Design review of the part built by this model. Coordinates are the model's own, in mm. Coordinates: 2 decimals unless noted, no trailing zeros. Loops run counter-clockwise (first coordinate to the right, second up) from the corner with the lowest first, then second, coordinate; pieces in that order, holes last. Notation, with made-up numbers: M -18.5,-37.5 L 6.5,-37.5 A12 ccw 6.5,-27.5 Z; hole C -33,-35.75 d8. An arc over 180 degrees is marked long. One line per item, written item: value.
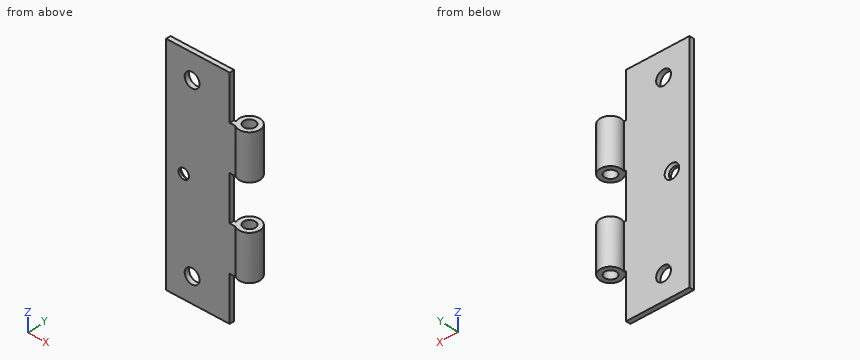
```python
from build123d import *

# Parameters (mm, degrees)
BOSS_EXTRUDE1_DEPTH                            = 15.24
SKETCH2_W                                      = 15.24
SKETCH2_H                                      = 1.5748
BOSS_EXTRUDE2_DEPTH                            = 0.254646985
SKETCH3_W                                      = 30.48
SKETCH3_H                                      = 1.5748
BOSS_EXTRUDE3_DEPTH                            = 21.866377542
SKETCH4_W                                      = 15.24
SKETCH4_H                                      = 1.5748
CUT_EXTRUDE1_DEPTH                             = 0.403377542
BOSS_EXTRUDE4_DEPTH                            = 15.24
SKETCH6_W                                      = 21.463
SKETCH6_H                                      = 1.5748
BOSS_EXTRUDE5_DEPTH                            = 15.24
SKETCH7_W                                      = 21.463
SKETCH7_H                                      = 1.5748
BOSS_EXTRUDE6_DEPTH                            = 15.24
SKETCH8_W                                      = 1.984375
SKETCH8_H                                      = 30.480025
M3_5_CLEARANCE_HOLE2_D                         = 3.96875
M3_5_CLEARANCE_HOLE2_DEPTH                     = 60.960025
CSK_FOR_M3_FLAT_HEAD_MACHINE_SCREW1_AT_2_COUNT = 2
CSK_FOR_M3_FLAT_HEAD_MACHINE_SCREW1_AT_2_PITCH = 59.436
CSK_FOR_M3_FLAT_HEAD_MACHINE_SCREW1_AT_3_COUNT = 2
CSK_FOR_M3_FLAT_HEAD_MACHINE_SCREW1_AT_3_PITCH = 29.851441177
SKETCH14_R                                     = 2.5
CUT_EXTRUDE2_DEPTH                             = 1.5748


with BuildPart() as part:
    # Sketch1 → Boss-Extrude1 (new body)
    with BuildSketch(Plane.XY.offset(-7.62)):
        with BuildLine():
            Line((-3.278975474, -1.376029012), (-3.278975474, -2.950829012))
            Line((-3.278975474, -2.950829012), (-1.984375, -2.950829012))
            ThreePointArc((-1.984375, -2.950829012), (2.746946179, 2.258190135), (-3.278975474, -1.376029012))
        make_face()
    extrude(amount=-BOSS_EXTRUDE1_DEPTH)

    # Sketch2 → Boss-Extrude2 (add)
    with BuildSketch(Plane.ZY.offset(3.278975474)):
        with Locations((-15.24, -2.163429012)):
            Rectangle(SKETCH2_W, SKETCH2_H)
    extrude(amount=BOSS_EXTRUDE2_DEPTH)

    # Sketch3 → Boss-Extrude3 (add)
    with BuildSketch(Plane.ZY.offset(3.533622458)):
        with Locations((-7.62, -2.163429012)):
            Rectangle(SKETCH3_W, SKETCH3_H)
    extrude(amount=BOSS_EXTRUDE3_DEPTH)

    # Sketch4 → Cut-Extrude1 (cut)
    with BuildSketch(Plane(origin=(-3.533622458, 0, 0), x_dir=(0, 0, -1), z_dir=(1, 0, 0))):
        with Locations((0, -2.163429012)):
            Rectangle(SKETCH4_W, SKETCH4_H)
    extrude(amount=-CUT_EXTRUDE1_DEPTH, mode=Mode.SUBTRACT)

    # Sketch5 → Boss-Extrude4 (add)
    with BuildSketch(Plane.XY.offset(7.62)):
        with BuildLine():
            Line((-25.4, -1.376029012), (-3.278975474, -1.376029012))
            ThreePointArc((-3.278975474, -1.376029012), (2.746946179, 2.258190135), (-1.984375, -2.950829012))
            Line((-1.984375, -2.950829012), (-25.4, -2.950829012))
            Line((-25.4, -2.950829012), (-25.4, -1.376029012))
        make_face()
    extrude(amount=BOSS_EXTRUDE4_DEPTH)

    # Sketch6 → Boss-Extrude5 (add)
    with BuildSketch(Plane.XY.offset(22.86)):
        with Locations((-14.6685, -2.163429012)):
            Rectangle(SKETCH6_W, SKETCH6_H)
    extrude(amount=BOSS_EXTRUDE5_DEPTH)

    # Sketch7 → Boss-Extrude6 (add)
    with BuildSketch(Plane(origin=(0, 0, -22.86), x_dir=(-1, 0, 0), z_dir=(0, 0, -1))):
        with Locations((14.6685, -2.163429012)):
            Rectangle(SKETCH7_W, SKETCH7_H)
    extrude(amount=BOSS_EXTRUDE6_DEPTH)

    # Sketch8 → M3.5 Clearance Hole1 (revolve, cut)
    with BuildSketch(Plane(origin=(0, 0, 7.62), x_dir=(0, 1, 0), z_dir=(1, 0, 0))):
        with Locations((0.9921875, 15.2400125)):
            Rectangle(SKETCH8_W, SKETCH8_H)
    revolve(axis=Axis((0, 0, 1.27), (0, 0, 1)), mode=Mode.SUBTRACT)

    # M3.5 Clearance Hole2
    with Locations(Plane(origin=(0, 0, -22.86), x_dir=(-1, 0, 0), z_dir=(0, 0, -1))):
        with Locations((0, 0)):
            Hole(M3_5_CLEARANCE_HOLE2_D / 2, depth=M3_5_CLEARANCE_HOLE2_DEPTH)

    # Sketch12 → CSK for M3 Flat Head Machine Screw1 (revolve, cut)
    with BuildSketch(Plane(origin=(-16.637, -1.376029012, -29.718), x_dir=(0, 0, 1), z_dir=(1, 0, 0))):
        Polygon((0, 0), (0, 2.179970988), (1.7526, 2.179970988), (1.7526, 0.7874), (2.437076377, 0), align=None)
    csk_for_m3_flat_head_machine_screw1 = revolve(axis=Axis((-16.637, 4.973970988, -29.718), (0, -1, 0)), mode=Mode.SUBTRACT)

    # CSK for M3 Flat Head Machine Screw1 at 2: CSK for M3 Flat Head Machine Screw1 ×2
    with Locations(*[(0, 0, i * CSK_FOR_M3_FLAT_HEAD_MACHINE_SCREW1_AT_2_PITCH) for i in range(1, CSK_FOR_M3_FLAT_HEAD_MACHINE_SCREW1_AT_2_COUNT)]):
        add(csk_for_m3_flat_head_machine_screw1, mode=Mode.SUBTRACT)

    # CSK for M3 Flat Head Machine Screw1 at 3: CSK for M3 Flat Head Machine Screw1 ×2
    with Locations(*[Vector(-0.094447701, 0, 0.995529825) * (i * CSK_FOR_M3_FLAT_HEAD_MACHINE_SCREW1_AT_3_PITCH) for i in range(1, CSK_FOR_M3_FLAT_HEAD_MACHINE_SCREW1_AT_3_COUNT)]):
        add(csk_for_m3_flat_head_machine_screw1, mode=Mode.SUBTRACT)

    # Sketch14 → Cut-Extrude2 (cut)
    with BuildSketch(Plane(origin=(0, -1.376029012, 0), x_dir=(1, 0, 0), z_dir=(0, 1, 0))):
        with Locations((-16.637, 29.718)):
            Circle(SKETCH14_R)
        with Locations((-16.637, -29.718)):
            Circle(SKETCH14_R)
    extrude(amount=-CUT_EXTRUDE2_DEPTH, mode=Mode.SUBTRACT)


solid = part.part
```
(1) We need section A-A on z = 0. State the section outline as (x, y) points.
Reply:
outline: M -25.4,-2.95 L -21.21,-2.95 L -21.21,-2.16 L -21.89,-1.38 L -25.4,-1.38 Z; M -17.7,-2.95 L -3.94,-2.95 L -3.94,-1.38 L -17.02,-1.38 L -17.7,-2.16 Z
(2) We need section D-D on z = -17. State the section outline as (x, y) points, then the cut area to 3 significant figures.
Reply:
outline: M -25.4,-2.95 L -1.98,-2.95 A3.56 ccw long -3.28,-1.38 L -25.4,-1.38 Z; hole C 0,0 d3.97
area: 63.0 mm2
(3) To check wall thickness, follow line 1 along X through (y, z) = (0, 19.25); line 2 along X through (y, z) = (-1.75, 29.5); line 3 along Z through (x, y) = (-3, 1.5). State the ranges of each line that lie inside material, in increasing order. Write a range as [from, to].
Reply:
line 1: x = [-3.56, -1.98], [1.98, 3.56]
line 2: x = [-25.4, -19.13], [-14.15, -3.94]
line 3: z = [-22.86, -7.62], [7.62, 22.86]
(4) We need section B-B on x = 0. State the section outline as (y, z) points, then the cut area to 3 significant figures.
Reply:
outline: M -3.56,-22.86 L -1.98,-22.86 L -1.98,-7.62 L -3.56,-7.62 Z; M -3.56,7.62 L -1.98,7.62 L -1.98,22.86 L -3.56,22.86 Z; M 1.98,-22.86 L 3.56,-22.86 L 3.56,-7.62 L 1.98,-7.62 Z; M 1.98,7.62 L 3.56,7.62 L 3.56,22.86 L 1.98,22.86 Z
area: 95.8 mm2
(5) Insertion check: pin 1 (1.3 mm diameter, centred on y = -2.5, z = 33, fed in from +X); pin 2 (3 mm diameter, centred on y = 1.5, z = -6.5, fed in from +X); pin 3 (2 mm diameter, centred on x = -1.5, y = -2.5, fed in from +Z); pin 4 (6 mm diameter, centred on x = -3, z = -19, fed in from +Y). Each pin has a flat end and moves straight along its axis. Give the tip position at first contact, or say it passes through.
Reply:
pin 1: stops at x = -3.94
pin 2: stops at x = 3.52
pin 3: stops at z = 22.86
pin 4: stops at y = 3.56
